For this review, take the finished solid that the model builds, in its own axes (mm). A direction names the side the tool comes from. Round coordinates to 2 decimals unless told otherwise and drop trailing zeros. Loops run counter-clockwise (first coordinate to the right, second up) from the corner with the lowest first, then second, coordinate; pieces in that order, holes last. Notation, with made-up numbers: (-13, 19) -> (46, 19) arc R22 cw to (46, 41) -> close; hole circle Ø1 at (2, 41.25). An arc over 180 degrees is marked (long way). One line per question, with ' | ' between items. Start each with the question number.
1. Draft analysis for pull direction Y (two halves, no side actions). For faces 1 (the face through (-23.724, -2.348, -4.144)), 2 (the face through (11.201, 2.36, -4.166)), 3 (the face through (11, 4.788, 0)), 4 (the face through (-23.724, 2.348, 4.144)), state which applies: pulls with the +Y half, pulls with the -Y half, needs draft (parallel to the pull), parting line crosses it, or undercut.
2. For pin 1 Ø4.5 at (x, z) = (11, 1) entering from -Y; pin 2 Ø1 at (x, z) = (-19.5, 3.5) entering from +Y; pin 3 Ø1 at (x, z) = (1, 1) entering from -Y, all flat-tipped, find the tip position at first contact; note any pin that passes through.
3. Wall thickness on line 1 along X through (y, z) = (-2, -6); line 2 along X through (y, z) = (-10, 8); line 3 along Z through (x, y) = (1, 5): over which ranges is each line inside the solid? List them lowest first.
4. For faces 5 (the face through (-24, -4.762, 0)), 6 (the face through (4.762, 0, 0)), 7 (the face through (-17.462, -5, 0)), list the 3-axis set-ups (+Z, -Z, +X, -X, +Y, -Y) from which the entire face can be reached by the end or side of a thin tool; tool diameter is ignored.
5. Consider section A-A (x = -19). Write out the cut boundary in (y, z), and give its area (3 significant figures).
```python
from build123d import *

# Parameters (mm, degrees)
F3_DEPTH = 12.7
F5_DEPTH = 12.7


with BuildPart() as f1:
    # F0 (on Front) → F1 (revolve)
    with BuildSketch(Plane.XZ):
        with BuildLine():
            Line((17.4625, 0), (17.4625, 10.998523))
            ThreePointArc((17.4625, 10.998523), (0, 20.6375), (-17.4625, 10.998523))
            Line((-17.4625, 10.998523), (-17.4625, 0))
            Line((-17.4625, 0), (17.4625, 0))
        make_face()
    revolve(axis=Axis((-1.484415, 0, 0), (1, 0, 0)))

    # F2 (on face) → F3 (cut)
    with BuildSketch(Plane.YZ.offset(17.4625)):
        Polygon((4.7879, -2.764295), (4.7879, 2.764295), (0, 5.528591), (-4.7879, 2.764295), (-4.7879, -2.764295), (0, -5.528591), align=None)
    extrude(amount=-F3_DEPTH, mode=Mode.SUBTRACT)

    # F4 (on face) → F5 (join)
    with BuildSketch(Plane(origin=(-17.4625, 0, 0), x_dir=(0, -1, 0), z_dir=(-1, 0, 0))):
        Polygon((4.7625, -2.749631), (4.7625, 2.749631), (0, 5.499261), (-4.7625, 2.749631), (-4.7625, -2.749631), (0, -5.499261), align=None)
    extrude(amount=F5_DEPTH)


solid = f1.part
```
Answer block:
1) face 1: pulls with the -Y half | face 2: undercut | face 3: undercut | face 4: pulls with the +Y half
2) pin 1: stops at y = -18.67 | pin 2: stops at y = 4.33 | pin 3: stops at y = -20.62
3) line 1: x = -17.46 to 17.46 | line 2: x = -16.18 to 16.18 | line 3: z = -20 to 20
4) face 5: +Z, -Z, -X, -Y | face 6: +X | face 7: -X
5) outline: (-4.76, -2.75) -> (0, -5.5) -> (4.76, -2.75) -> (4.76, 2.75) -> (0, 5.5) -> (-4.76, 2.75) -> close | area: 78.6 mm2
